For this review, take the finished solid that the model builds, in its own axes (mm). A direction names the side the tool comes from. Round coordinates to 2 decimals unless told otherwise and drop trailing zeros. Write each loop counter-clockwise with the first axis right and the second up, starting at its lowest first coordinate (ties: lowest second). Pieces come first, ordered by that corner, then holes.
from build123d import *

# Parameters (mm, degrees)
BOSS_EXTRUDE1_DEPTH      = 3
BOSS_EXTRUDE1_DEPTH_BACK = 1
SKETCH1_W                = 69
SKETCH1_H                = 22
SKETCH2_W                = 13
SKETCH2_H                = 10
BOSS_EXTRUDE2_DEPTH      = 9.5
CUT_EXTRUDE1_DEPTH       = 10
FILLET1_R                = 2
FILLET2_R                = 1.5
CHAMFER1_SIZE            = 3
FILLET3_R                = 1.5
FILLET4_R                = 2


with BuildPart() as part:
    # Sketch1 → Boss-Extrude1 (new, two sides: drawn at the far end of the back side and taken through both)
    with BuildSketch(Plane(origin=(0, 0, 0), x_dir=(1, 0, 0), z_dir=(0, 1, 0)).offset(-BOSS_EXTRUDE1_DEPTH_BACK)):
        Rectangle(SKETCH1_W, SKETCH1_H)
    extrude(amount=BOSS_EXTRUDE1_DEPTH + BOSS_EXTRUDE1_DEPTH_BACK)

    # Sketch2 → Boss-Extrude2 (add)
    with BuildSketch(Plane(origin=(0, 3, 0), x_dir=(1, 0, 0), z_dir=(0, 1, 0))):
        with Locations((-28, -6)):
            Rectangle(SKETCH2_W, SKETCH2_H)
        with Locations((28, -6)):
            Rectangle(SKETCH2_W, SKETCH2_H)
    extrude(amount=BOSS_EXTRUDE2_DEPTH)

    # Sketch3 → Cut-Extrude1 (cut)
    with BuildSketch(Plane(origin=(-21.5, 0, 0), x_dir=(0, 0, -1), z_dir=(1, 0, 0))):
        Polygon((-1, 3), (-1, 8.5), (-5, 8.5), align=None)
    extrude(amount=-CUT_EXTRUDE1_DEPTH, mode=Mode.SUBTRACT)

    # Fillet1
    fillet1_edges = [part.edges().sort_by_distance(p)[0] for p in [
        (34.5, 12.5, 6),
        (21.5, 12.5, 6),
    ]]
    fillet(fillet1_edges, radius=FILLET1_R)

    # Fillet2
    fillet2_edges = [part.edges().sort_by_distance(p)[0] for p in [
        (28, 12.5, 1),
        (21.5, 6.75, 1),
        (34.5, 6.75, 1),
        (33.914213562, 11.914213562, 1),
        (22.085786438, 11.914213562, 1),
    ]]
    fillet(fillet2_edges, radius=FILLET2_R)

    # Chamfer1
    chamfer1_edges = [part.edges().sort_by_distance(p)[0] for p in [
        (-21.5, 10.5, 1),
        (-21.5, 12.5, 6),
    ]]
    chamfer(chamfer1_edges, length=CHAMFER1_SIZE)

    # Fillet3
    fillet3_edges = [part.edges().sort_by_distance(p)[0] for p in [
        (-34.5, 7.75, 1),
        (-29.5, 12.5, 1),
    ]]
    fillet(fillet3_edges, radius=FILLET3_R)

    # Fillet4
    # the kernel refuses this fillet: 2 mm, written as the material it takes off along each edge
    with BuildSketch(Plane(origin=(-32.5, 10.5, 1), x_dir=(-1, 0, 0), z_dir=(0, -1, 0))) as fillet4_piece_1:
        with BuildLine():
            CenterArc((0.5, -1.5), 1.5, 0, 90)
            Line((2, -1.5), (2, 0))
            Line((2, 0), (0.5, 0))
        make_face()
    revolve(axis=Axis((-32.5, 10.5, 1), (0, 0, -1)), revolution_arc=90, mode=Mode.SUBTRACT)
    with BuildSketch(Plane(origin=(-34.5, 12.5, 1), x_dir=(0, -1, 0), z_dir=(0, 0, 1))) as fillet4_piece_2:
        with BuildLine():
            CenterArc((FILLET4_R, FILLET4_R), FILLET4_R, 180, 90)
            Line((0, FILLET4_R), (0, 0))
            Line((0, 0), (FILLET4_R, 0))
        make_face()
    extrude(amount=15, mode=Mode.SUBTRACT)


solid = part.part
(1) We need section A-A, the plane y = 5. Give the boundary of the cut face in (x, z).
Geometry check:
outline: (-34.5, 2.5) arc R1.5 ccw to (-33, 1) - (-31.5, 1) - (-31.5, 2.45) - (-21.5, 2.45) - (-21.5, 11) - (-34.5, 11) - close; (21.5, 2.5) arc R1.5 ccw to (23, 1) - (33, 1) arc R1.5 ccw to (34.5, 2.5) - (34.5, 11) - (21.5, 11) - close
(2) For faces 1 (the face through (34.07, 6.7, 1.45)), 2 (the face through (0, 3, -3)), 3 (the face through (-30, 9, 1)), 4 (the face through (-34.05, 6.8, 1.43)), 5 (the face through (-21.5, 6, 7)), list the 3-axis set-ups (+Z, -Z, +X, -X, +Y, -Y) from which the entire face can be reached by the end or side of a thin tool; tool diameter is ignored.
Geometry check:
face 1: -Z, +X, +Y
face 2: -Z, +Y
face 3: -Z, +X, -X, +Y
face 4: -Z, -X, +Y
face 5: +Z, -Z, +Y
(3) For pin 1 Ø4 at (x, y) = (29.5, 5.5) entering from -Z; pin 2 Ø6 at (y, z) = (8, -1) entering from +X; pin 3 Ø6 at (y, z) = (11, 7.5) entering from +X; pin 4 Ø1.5 at (x, z) = (7.5, 5) entering from +Y, all flat-tipped, find the tip position at first contact; note any pin that passes through.
Geometry check:
pin 1: stops at z = 1
pin 2: stops at x = 34.41
pin 3: stops at x = 34.5
pin 4: stops at y = 3
(4) Mouldability with a two-part tool opening along Y and no side actions: class faces 6 (the face through (-28.22, 12.05, 1.43)), 7 (the face through (-31.5, 7, 2)), 8 (the face through (-0.5, 2.7, 11)) as pulls with the +Y half, pulls with the -Y half, needs draft (parallel to the pull), parting line crosses it, or undercut.
Geometry check:
face 6: pulls with the +Y half
face 7: undercut
face 8: needs draft
(5) We need section B-B, the plane z = 6.75. Give the boundary of the cut face in (x, y), and give its area (3 significant figures).
Geometry check:
outline: (-34.5, -1) - (34.5, -1) - (34.5, 10.5) arc R2 ccw to (32.5, 12.5) - (23.5, 12.5) arc R2 ccw to (21.5, 10.5) - (21.5, 3) - (-21.5, 3) - (-21.5, 9.5) - (-24.5, 12.5) - (-32.5, 12.5) arc R2 ccw to (-34.5, 10.5) - close
area: 516 mm2
(6) We need section C-C, the plane x = -16. Give the boundary of the cut face in (y, z).
Geometry check:
outline: (-1, -11) - (3, -11) - (3, 11) - (-1, 11) - close
(7) For line 1 along X through (y, z) = (8, 9.75); line 2 along Y through (x, z) = (-8, -0.75); line 3 along Z through (x, y) = (23.5, 7.5), list the stretches that pass through material, from the lowest coordinate up.
Geometry check:
line 1: x = -34.5 to -21.5, 21.5 to 34.5
line 2: y = -1 to 3
line 3: z = 1 to 11
(8) We need section D-D, the plane z = -7.5. Give the boundary of the cut face in (x, y), and give its area (3 significant figures).
Geometry check:
outline: (-34.5, -1) - (34.5, -1) - (34.5, 3) - (-34.5, 3) - close
area: 276 mm2
